from build123d import *

# Parameters (mm, degrees)
BOSS_EXTRUDE1_DEPTH         = 3.175
CHAMFER1_SIZE               = 3
TAP_DRILL_FOR_M2X0_4_TAP1_D = 1.6
M2_CLEARANCE_HOLE1_D        = 2.2


with BuildPart() as part:
    # Sketch1 → Boss-Extrude1 (new body)
    with BuildSketch(Plane.XY):
        Polygon((6, 27.65), (-6, 27.65), (-6, 3.175), (-10.25, 3.175), (-10.25, 0), (-1.5, 0), (-1.5, 22.8), (-0.95, 26.45), (0.95, 26.45), (1.5, 22.8), (1.5, 0), (10.25, 0), (10.25, 3.175), (6, 3.175), align=None)
    extrude(amount=BOSS_EXTRUDE1_DEPTH)

    # Chamfer1
    chamfer1_edges = [part.edges().sort_by_distance(p)[0] for p in [
        (-6, 27.65, 1.5875),
        (6, 27.65, 1.5875),
    ]]
    chamfer(chamfer1_edges, length=CHAMFER1_SIZE)

    # Tap Drill for M2x0.4 Tap1 (through all)
    with Locations(Plane(origin=(6, 0, 0), x_dir=(0, 0, -1), z_dir=(1, 0, 0))):
        with Locations((-1.5875, 15.3)):
            Hole(TAP_DRILL_FOR_M2X0_4_TAP1_D / 2)

    # M2 Clearance Hole1 (through all)
    with Locations(Plane.XY.offset(3.175)):
        with Locations((-8, 1.5875), (8, 1.5875)):
            Hole(M2_CLEARANCE_HOLE1_D / 2)


solid = part.part
Geometry check sheet. Reference: the model listing, model coordinates, mm. A direction names the side the tool comes from. Give positions to 0.01 mm unless a question says otherwise; leave off trailing zeros. Loops run counter-clockwise (first coordinate to the right, second up) from the corner with the lowest first, then second, coordinate; pieces in that order, holes last. Notation, with made-up numbers: M 37,16.5 L 56,16.5 A28 ccw 56,38.5 Z; hole C -30.75,1.5 d7. An arc over 180 degrees is marked long. Write each question's results on one line, items separated by ' | '.
1) Tool access check on faces 1 (the face through (8, 3.175, 2)), 2 (the face through (-2, 14, 3.175)), 3 (the face through (1.5, 12, 2)), 4 (the face through (-8, 3.175, 2)). Record the directions out of +Z, -Z, +X, -X, +Y, -Y that give a thin tool (end or side, any length) a straight path to the whole face; none if there is none.
Answers follow:
face 1: +Z, -Z, +X, +Y | face 2: +Z, +X, -X, +Y, -Y | face 3: +Z, -Z, -Y | face 4: +Z, -Z, -X, +Y
2) Gauge pin test, flat ends, axial feed: pin 1 (1.4 mm diameter, centred on y = 15.3, z = 1.59, fed in from +X); pin 2 (1.6 mm diameter, centred on x = 8.5, z = 2.5, fed in from +Y) (3 decimals); pin 3 (1 mm diameter, centred on y = 9.5, z = 1.5, fed in from -X); pin 4 (1 mm diameter, centred on y = 8.5, z = 2, fed in from +X). Record the tip position at first contact, or that the pin passes through.
Answers follow:
pin 1: through | pin 2: y = 3.175 | pin 3: x = -6 | pin 4: x = 6
3) Section check D-D, the plane y = 8.75. Record the boundary of the cut face in (x, z) (3 decimals), plus the area to 3 significant figures.
Answers follow:
outline: M -6,0 L -1.5,0 L -1.5,3.175 L -6,3.175 Z; M 1.5,0 L 6,0 L 6,3.175 L 1.5,3.175 Z | area: 28.6 mm2
4) Section check A-A, the plane y = 15.3. Record the boundary of the cut face in (x, z) (1 decimal), plus the area to 3 significant figures.
Answers follow:
outline: M -6,0 L -1.5,0 L -1.5,0.8 L -6,0.8 Z; M -6,2.4 L -1.5,2.4 L -1.5,3.2 L -6,3.2 Z; M 1.5,0 L 6,0 L 6,0.8 L 1.5,0.8 Z; M 1.5,2.4 L 6,2.4 L 6,3.2 L 1.5,3.2 Z | area: 14.2 mm2
5) Thickness scan on line 1 (X direction, y = 1.5, z = 1.9); line 2 (Y direction, x = -8, z = 0.8) (1 decimal); line 3 (X direction, y = 11.75, z = 1.9). Record the ranges inside material, lowest first.
Answers follow:
line 1: -10.25 to -9.1, -6.9 to -1.5, 1.5 to 6.9, 9.1 to 10.25 | line 2: 0 to 0.5, 2.7 to 3.2 | line 3: -6 to -1.5, 1.5 to 6
6) Release check for a two-part mould opening along Y. For faces 5 (the face through (-1.5, 11, 2)), 6 (the face through (-1.23, 24.6, 1.57)), 7 (the face through (-3.782, 16.093, 1.483)), 8 (the face through (0, 27.65, 2)) record: +Y half, -Y half, draft (parallel to the pull), parting line (faces both ways), or undercut.
Answers follow:
face 5: draft | face 6: -Y half | face 7: undercut | face 8: +Y half
7) Section check B-B, the plane x = -8. Record the boundary of the cut face in (y, z) (1 decimal).
Answers follow:
outline: M 0,0 L 0.5,0 L 0.5,3.2 L 0,3.2 Z; M 2.7,0 L 3.2,0 L 3.2,3.2 L 2.7,3.2 Z
